For this review, take the finished solid that the model builds, in its own axes (mm). Round coordinates to 2 decimals unless told otherwise and drop trailing zeros. Order: outer loops, then holes, each group sorted by start corner. A loop starts at its lowest first (then second) coordinate and runs counter-clockwise, first axis right, second up. Notation, with made-up numbers: M 42.25,15.25 L 87.25,15.25 A33 cw 87.25,51.25 Z; hole C -29,67 d9. An arc over 180 degrees is marked long. Put each result on its own line as item: value.
from build123d import *

# Parameters (mm, degrees)
SKETCH1_R           = 3.175
SKETCH1_R_2         = 1.397
BOSS_EXTRUDE1_DEPTH = 3.175


with BuildPart() as part:
    # Sketch1 → Boss-Extrude1 (new body)
    # profile 1 of 5: a face of its own
    with BuildSketch(Plane.XY):
        with BuildLine():
            Line((0, 58.42), (0, 53.213))
            Line((0, 53.213), (1.8034, 53.213))
            Line((1.8034, 53.213), (1.8034, 6.35))
            Line((1.8034, 6.35), (0, 6.35))
            Line((0, 6.35), (0, 6.731))
            Line((0, 6.731), (-3.556, 6.731))
            ThreePointArc((-3.556, 6.731), (-1.31093597, 5.80106403), (-0.381, 3.556))
            ThreePointArc((-0.381, 3.556), (-3.556, 0.381), (-6.731, 3.556))
            Line((-6.731, 3.556), (-6.731, 0))
            Line((-6.731, 0), (-10.287, 0))
            Line((-10.287, 0), (-10.287, -1.8034))
            Line((-10.287, -1.8034), (-45.847, -1.8034))
            Line((-45.847, -1.8034), (-45.847, 0))
            Line((-45.847, 0), (-49.403, 0))
            Line((-49.403, 0), (-49.403, 3.556))
            ThreePointArc((-49.403, 3.556), (-54.82306403, 1.31093597), (-52.578, 6.731))
            Line((-52.578, 6.731), (-56.134, 6.731))
            Line((-56.134, 6.731), (-56.134, 6.35))
            Line((-56.134, 6.35), (-57.9374, 6.35))
            Line((-57.9374, 6.35), (-57.9374, 53.213))
            Line((-57.9374, 53.213), (-56.134, 53.213))
            Line((-56.134, 53.213), (-56.134, 58.42))
            Line((-56.134, 58.42), (-52.578, 58.42))
            ThreePointArc((-52.578, 58.42), (-55.753, 61.595), (-52.578, 64.77))
            Line((-52.578, 64.77), (-57.9374, 64.77))
            ThreePointArc((-57.9374, 64.77), (-59.733451224, 64.026051224), (-60.4774, 62.23))
            Line((-60.4774, 62.23), (-60.4774, -1.8034))
            ThreePointArc((-60.4774, -1.8034), (-59.733451224, -3.599451224), (-57.9374, -4.3434))
            Line((-57.9374, -4.3434), (1.8034, -4.3434))
            ThreePointArc((1.8034, -4.3434), (3.599451224, -3.599451224), (4.3434, -1.8034))
            Line((4.3434, -1.8034), (4.3434, 62.23))
            ThreePointArc((4.3434, 62.23), (3.599451224, 64.026051224), (1.8034, 64.77))
            Line((1.8034, 64.77), (-3.556000021, 64.77))
            ThreePointArc((-3.556000021, 64.77), (-1.310935977, 63.840064038), (-0.381, 61.595))
            ThreePointArc((-0.381, 61.595), (-1.31093597, 59.34993597), (-3.556, 58.42))
            Line((-3.556, 58.42), (0, 58.42))
        make_face()
    # profile 2 of 5: a face of its own
    with BuildSketch(Plane.XY):
        with Locations((-52.578, 61.595)):
            Circle(SKETCH1_R)
        with Locations((-52.578, 61.595)):
            Circle(SKETCH1_R_2, mode=Mode.SUBTRACT)
    # profile 3 of 5: a face of its own
    with BuildSketch(Plane.XY):
        with Locations((-3.556, 61.595)):
            Circle(SKETCH1_R)
        with Locations((-3.556, 61.595)):
            Circle(SKETCH1_R_2, mode=Mode.SUBTRACT)
    # profile 4 of 5: a face of its own
    with BuildSketch(Plane.XY):
        with Locations((-52.578, 3.556)):
            Circle(SKETCH1_R)
        with Locations((-52.578, 3.556)):
            Circle(SKETCH1_R_2, mode=Mode.SUBTRACT)
    # profile 5 of 5: a face of its own
    with BuildSketch(Plane.XY):
        with Locations((-3.556, 3.556)):
            Circle(SKETCH1_R)
        with Locations((-3.556, 3.556)):
            Circle(SKETCH1_R_2, mode=Mode.SUBTRACT)
    extrude(amount=BOSS_EXTRUDE1_DEPTH)


solid = part.part
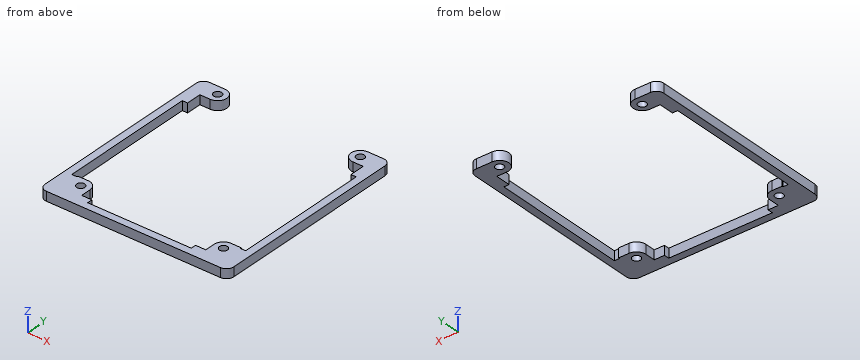
(1) Add section C-C on z = 1.85. State how many separate pieces and enclosed holes the cut face has, then the cut area to 3 significant figures.
A:
separate pieces: 1
enclosed holes: 4
area: 744 mm2
(2) To check wall thickness, follow L1, parallel to X at y = 28, z = 0.8; L2, parallel to X at y = 55.5, z = 2.5; L3, parallel to Y at x = -55.5, z = 2.85. State the ranges of each line that lie inside material, in increasing order.
A:
L1: x = -60.48 to -57.94, 1.8 to 4.34
L2: x = -60.48 to -56.13, 0 to 4.34
L3: y = -4.34 to 6.73, 58.42 to 64.77
(3) Add section B-B on x = -9. Give the boundary of the cut face in (y, z) (3 decimals), then the cut area to 3 significant figures.
A:
outline: M -4.343,0 L 0,0 L 0,3.175 L -4.343,3.175 Z
area: 13.8 mm2
(4) Insertion check: pin 1 Ø2.5 at (x, y) = (-52.578, 3.556) entering from +Z; pin 2 Ø1.6 at (x, z) = (-9, 2) entering from +Y; pin 3 Ø3.5 at (x, y) = (-3.556, 61.595) entering from +Z (3 decimals). Each pin has a flat end and moves straight along its axis. Give the tip position at first contact, or say it passes through.
A:
pin 1: passes through
pin 2: stops at y = 0
pin 3: stops at z = 3.175
(5) Add section D-D on x = -35.5. Give the boundary of the cut face in (y, z) (3 decimals).
A:
outline: M -4.343,0 L -1.803,0 L -1.803,3.175 L -4.343,3.175 Z
(6) Add section A-A on y = 50.5. Give the boundary of the cut face in (x, z) (3 decimals), then the cut area to 3 significant figures.
A:
outline: M -60.477,0 L -57.937,0 L -57.937,3.175 L -60.477,3.175 Z; M 1.803,0 L 4.343,0 L 4.343,3.175 L 1.803,3.175 Z
area: 16.1 mm2
